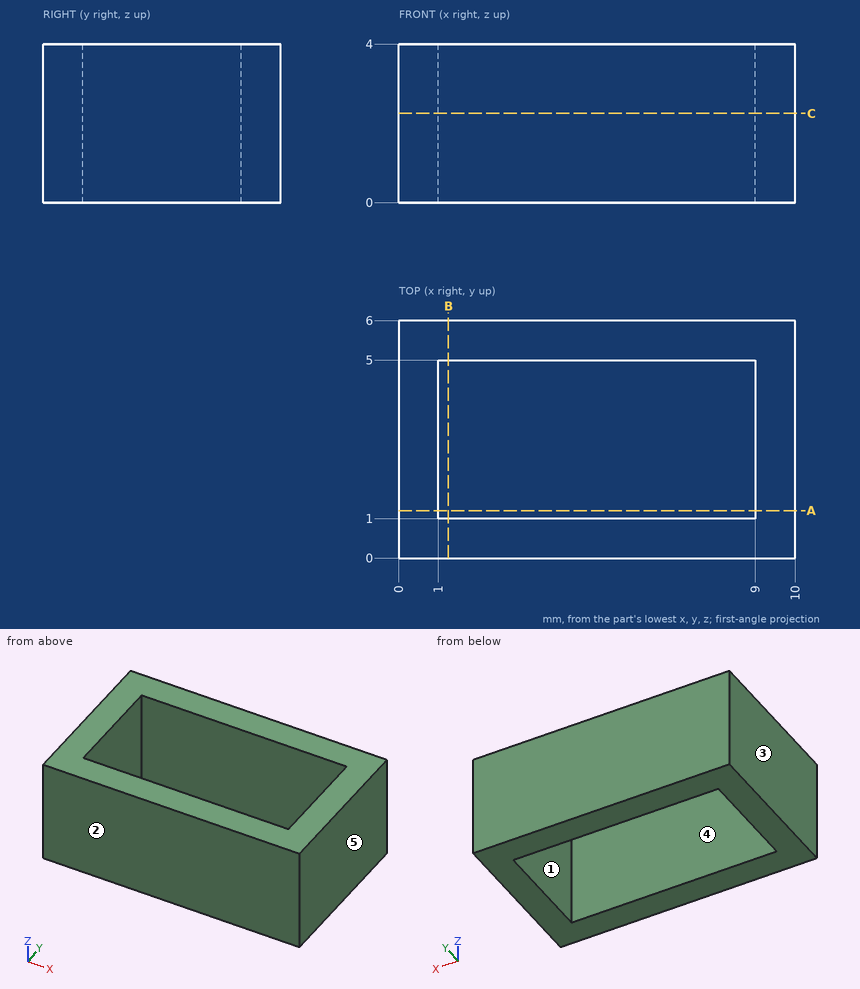
Part print with two shaded views. Sizes in mm from the minimum x, y, z corner. A direction names the side the tool comes from. Coordinates: 2 decimals unless noted, no trailing zeros. Order: outer loops, then holes, each group sorted by start corner. A loop starts at its lowest first (then second) coordinate and runs counter-clockwise, first axis right, second up. Notation, with made-up numbers: M 52.5,51.25 L 102.5,51.25 A25 cw 102.5,84.25 Z; hole C 59.25,42.25 d9. An arc over 180 degrees is marked long. Use a Markdown table: item, result.
(1) Tool access for the marked faces 4 and 5: list every direction of +Z, -Z, +X, -X, +Y, -Y with a clear straight run to the whole face (end or side of a thin tool).
A:
| item | result |
|---|---|
| face 4 | +Z, -Z |
| face 5 | +Z, -Z, +X, +Y, -Y |
(2) Cut at B-B on x = 1.25. Write the cut outline in (y, z), then the cut area to 3 significant figures.
A:
| item | result |
|---|---|
| outline | M 0,0 L 1,0 L 1,4 L 0,4 Z; M 5,0 L 6,0 L 6,4 L 5,4 Z |
| area | 8.00 mm^2 |
(3) Cut at C-C on z = 2.25. Write the cut outline in (x, y).
A:
| item | result |
|---|---|
| outline | M 0,0 L 10,0 L 10,6 L 0,6 Z; hole M 1,1 L 9,1 L 9,5 L 1,5 Z |
(4) Pull direction X, two halves, no side cores. Call the marked faces 1, 2 and 3: released by +X, released by -X, zero draft, split by the parting line, or undercut.
A:
| item | result |
|---|---|
| face 1 | undercut |
| face 2 | zero draft |
| face 3 | released by -X |
(5) Cut at A-A on y = 1.2. Write the cut outline in (x, z).
A:
| item | result |
|---|---|
| outline | M 0,0 L 1,0 L 1,4 L 0,4 Z; M 9,0 L 10,0 L 10,4 L 9,4 Z |
(6) Probe L1, parallel to X at y = 2.2, z = 1.1; L2, parallel to Y at x = 7.5, z = 3. List the from-to ranges inside material, lowest first.
A:
| item | result |
|---|---|
| L1 | x = 0 to 1, 9 to 10 |
| L2 | y = 0 to 1, 5 to 6 |
